Can you work these out from the model? Positions are in its coordinate system, mm. A direction names the side the tool comes from. Coordinates: 2 decimals unless noted, no trailing zeros. Order: outer loops, then holes, each group sorted by start corner. A loop starts at its lowest first (then second) coordinate and runs counter-clockwise, first axis right, second up.
```python
from build123d import *

# Parameters (mm, degrees)
PAD011_DEPTH    = 10
PAD012_DEPTH    = 6
POCKET014_DEPTH = 221.3994809485
SKETCH029_R     = 2
SKETCH029_R_2   = 4.6
POCKET015_DEPTH = 10.001
SKETCH030_R     = 4
POCKET016_DEPTH = 3
SKETCH031_R     = 15
POCKET017_DEPTH = 8.5


with BuildPart() as part:
    # Sketch025 → Pad011 (new body)
    with BuildSketch(Plane.XY.offset(70.1)):
        with BuildLine():
            Line((-27.5, 25.5), (-27.5, -25.5))
            ThreePointArc((-27.5, -25.5), (-26.9142135624, -26.9142135624), (-25.5, -27.5))
            Line((-25.5, -27.5), (25.5, -27.5))
            ThreePointArc((25.5, -27.5), (26.9142135624, -26.9142135624), (27.5, -25.5))
            Line((27.5, -25.5), (27.5, 25.5))
            ThreePointArc((27.5, 25.5), (26.9142135624, 26.9142135624), (25.5, 27.5))
            Line((25.5, 27.5), (-25.5, 27.5))
            ThreePointArc((-25.5, 27.5), (-26.9142135624, 26.9142135624), (-27.5, 25.5))
        make_face()
    extrude(amount=-PAD011_DEPTH)

    # Sketch027 → Pad012 (join)
    with BuildSketch(Plane.XY.offset(60.1)):
        Polygon((-19.9456135517, -6.25), (-16.38, -7.83), (-21.4441025641, -19.2582485631), (-25.0097161158, -17.6782485631), align=None)
    pad012 = extrude(amount=-PAD012_DEPTH)

    # Sketch028 (on Face12 of Pad012) → Pocket014 (cut, through all)
    with BuildSketch(Plane(origin=(-10.6527063441, -24.0401481662, 0), x_dir=(0.914259885, -0.4051282051, 0), z_dir=(-0.4051282051, -0.914259885, 0))):
        with BuildLine():
            ThreePointArc((-11.8034230709, 54.1), (-13.7534230709, 56.05), (-15.7034230709, 54.1))
            Line((-11.8034230709, 54.1), (-15.7034230709, 54.1))
        make_face()
    pocket014 = extrude(amount=-POCKET014_DEPTH, mode=Mode.SUBTRACT)

    # Mirrored001: Pad012, Pocket014 across YZ
    add(pad012.mirror(Plane.YZ))
    add(pocket014.mirror(Plane.YZ), mode=Mode.SUBTRACT)

    # Sketch029 → Pocket015 (cut, through all)
    with BuildSketch(Plane.XY.offset(60.1)):
        with Locations((19.5, 19.5)):
            Circle(SKETCH029_R)
        with Locations((-19.5, 19.5)):
            Circle(SKETCH029_R)
        with Locations((-13.5, -19.5)):
            Circle(SKETCH029_R)
        with Locations((13.5, -19.5)):
            Circle(SKETCH029_R)
        Circle(SKETCH029_R_2)
        with BuildLine():
            ThreePointArc((-12.595, -8.1465314705), (0, -15), (12.595, -8.1465314705))
            Line((-12.595, -8.1465314705), (12.595, -8.1465314705))
        make_face()
    extrude(amount=POCKET015_DEPTH, mode=Mode.SUBTRACT)

    # Sketch030 → Pocket016 (cut)
    with BuildSketch(Plane.XY.offset(70.1)):
        with Locations((13.5, -19.5)):
            Circle(SKETCH030_R)
        with Locations((-13.5, -19.5)):
            Circle(SKETCH030_R)
        with Locations((-19.5, 19.5)):
            Circle(SKETCH030_R)
        with Locations((19.5, 19.5)):
            Circle(SKETCH030_R)
    extrude(amount=-POCKET016_DEPTH, mode=Mode.SUBTRACT)

    # Sketch031 → Pocket017 (cut)
    with BuildSketch(Plane.XY.offset(60.1)):
        Circle(SKETCH031_R)
    extrude(amount=POCKET017_DEPTH, mode=Mode.SUBTRACT)


solid = part.part
```
1. I'm going to push flat-ended pins straight in: pin 1 (10.5 mm diameter, centred on x = 0, y = 0, fed in from -Z); pin 2 (2.5 mm diameter, centred on x = 20, y = 20.5, fed in from +Z); pin 3 (6.5 mm diameter, centred on x = 19.5, y = 19.5, fed in from -Z); pin 4 (3.5 mm diameter, centred on x = 19.5, y = 19.5, fed in from -Z). Where does each tip first touch, or does it pass through?
Completed:
pin 1: stops at z = 68.6
pin 2: stops at z = 67.1
pin 3: stops at z = 60.1
pin 4: passes through
2. On a 3-axis mill with a long thin cutter (end or side, diameter ignored), from which of +Z, -Z, +X, -X, +Y, -Y can I reach the whole of each face in a straight line? I mean faces 1 (the flat face through (3, 4, 68.6)), 2 (the flat face through (-11.8, -21.2, 67.1)), 3 (the flat face through (-23.2, -18.48, 57.81)), 4 (the flat face through (0, -8.147, 69)). Say none if no direction works.
Completed:
face 1: -Z
face 2: +Z
face 3: -Z, -X, -Y
face 4: +Z, -Z
3. Please list where these lines run through material, in increasing order: probe 1 along X at (y, z) = (-19.5, 62.25); probe 2 along X at (y, z) = (19.5, 62); probe 3 along Y at (x, z) = (19.5, 63.5).
Completed:
probe 1: x = -27.5 to -15.5, -11.5 to 11.5, 15.5 to 27.5
probe 2: x = -27.5 to -21.5, -17.5 to 17.5, 21.5 to 27.5
probe 3: y = -27.5 to 17.5, 21.5 to 27.5
4. Imagine slicing it at C-C on x = 0. Please give me the cut outline in (y, z), then the cut area to 3 significant figures.
Completed:
outline: (-27.5, 60.1) - (-15, 60.1) - (-15, 70.1) - (-27.5, 70.1) - close; (-8.15, 68.6) - (-4.6, 68.6) - (-4.6, 70.1) - (-8.15, 70.1) - close; (4.6, 68.6) - (15, 68.6) - (15, 60.1) - (27.5, 60.1) - (27.5, 70.1) - (4.6, 70.1) - close
area: 271 mm2
5. Imagine slicing it at A-A on z = 57.75. Please give me the cut outline in (x, y).
Completed:
outline: (-25.01, -17.68) - (-21.44, -19.26) - (-16.38, -7.83) - (-19.95, -6.25) - close; (16.38, -7.83) - (21.44, -19.26) - (25.01, -17.68) - (19.95, -6.25) - close
6. Imagine slicing it at D-D on x = 13.5. Please give me the cut outline in (y, z), then the cut area to 3 significant figures.
Completed:
outline: (-27.5, 60.1) - (-21.5, 60.1) - (-21.5, 67.1) - (-23.5, 67.1) - (-23.5, 70.1) - (-27.5, 70.1) - close; (-17.5, 60.1) - (-6.54, 60.1) - (-6.54, 68.6) - (6.54, 68.6) - (6.54, 60.1) - (27.5, 60.1) - (27.5, 70.1) - (-15.5, 70.1) - (-15.5, 67.1) - (-17.5, 67.1) - close
area: 387 mm2
7. Thinking about a two-plate mould opening in Y: for faces 5 (the flat face through (-27.5, 0, 65)), 6 (the cylindrical face through (18.979, 23.466, 68.621)), 7 (the flat face through (0, -27.5, 65)), which applies, pulls with the +Y half, pulls with the -Y half, needs draft (parallel to the pull), parting line crosses it, or undercut?
Completed:
face 5: needs draft
face 6: undercut
face 7: pulls with the -Y half
8. Imagine slicing it at B-B on y = 19.5. Please give me the cut outline in (x, z), then the cut area to 3 significant figures.
Completed:
outline: (-27.5, 60.1) - (-21.5, 60.1) - (-21.5, 67.1) - (-23.5, 67.1) - (-23.5, 70.1) - (-27.5, 70.1) - close; (-17.5, 60.1) - (17.5, 60.1) - (17.5, 67.1) - (15.5, 67.1) - (15.5, 70.1) - (-15.5, 70.1) - (-15.5, 67.1) - (-17.5, 67.1) - close; (21.5, 60.1) - (27.5, 60.1) - (27.5, 70.1) - (23.5, 70.1) - (23.5, 67.1) - (21.5, 67.1) - close
area: 446 mm2
